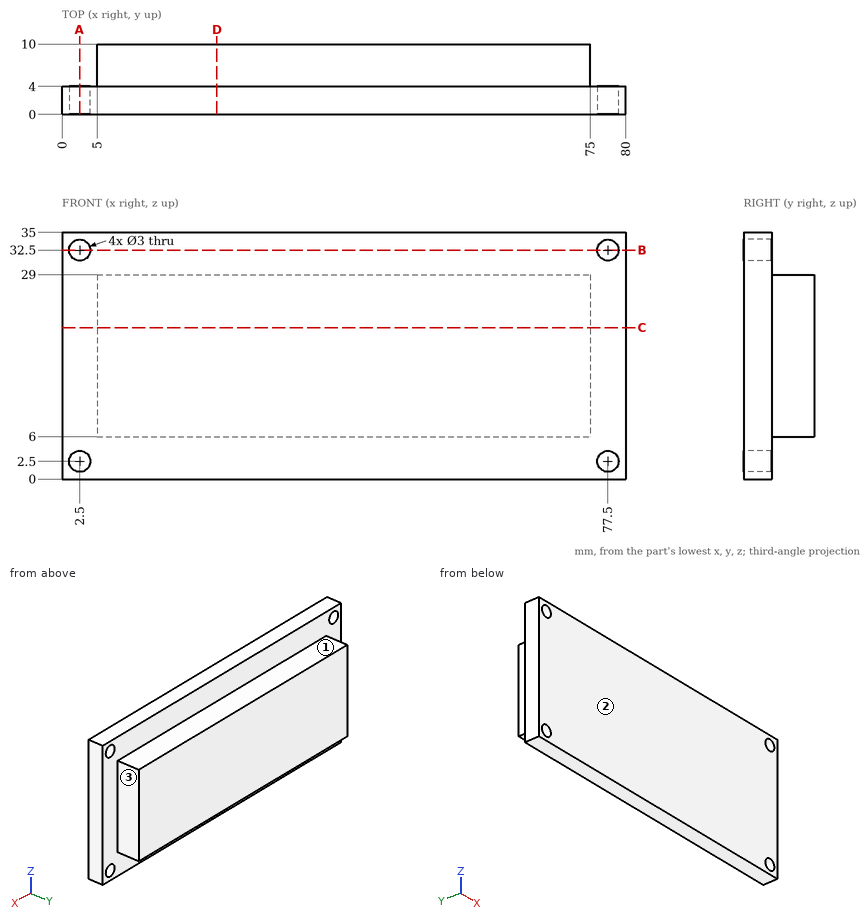
Print and shaded views of the part. All mm, measured from the part's lowest x, y and z. A direction names the side the tool comes from. Give positions to 0.01 mm unless a question says otherwise; leave off trailing zeros. Order: outer loops, then holes, each group sorted by start corner. A loop starts at its lowest first (then second) coordinate and runs counter-clockwise, first axis right, second up. Notation, with made-up numbers: (84, -14) - (136, -14) arc R18 cw to (136, 10) - close; hole circle Ø4 at (68.25, -15.5). An arc over 180 degrees is marked (long way). One line per item, written item: value.
Item 1: Slice it at D-D (x = 22). List the corners of the cut face in (y, z), then the cut area to 3 significant figures.
Response values:
outline: (0, 0) - (4, 0) - (4, 6) - (10, 6) - (10, 29) - (4, 29) - (4, 35) - (0, 35) - close
area: 278 mm2
Item 2: Slice it at A-A (x = 2.5). List the corners of the cut face in (y, z).
Response values:
outline: (0, 0) - (4, 0) - (4, 1) - (0, 1) - close; (0, 4) - (4, 4) - (4, 31) - (0, 31) - close; (0, 34) - (4, 34) - (4, 35) - (0, 35) - close
Item 3: Pin check, flat tips, straight feed: pin 1 Ø3.5 at (x, z) = (77.5, 32.5) entering from +Y; pin 2 Ø1 at (x, y) = (54.5, 6.5) entering from -Z; pin 3 Ø2.5 at (x, z) = (2.5, 2.5) entering from -Y; pin 4 Ø4 at (x, y) = (23, 7.5) entering from +Z. Stop position of each tip, or through.
Response values:
pin 1: y = 4
pin 2: z = 6
pin 3: through
pin 4: z = 29
Item 4: Tool access for the marked faces 1, 2 and 3: list every direction of +Z, -Z, +X, -X, +Y, -Y with a clear straight run to the whole face (end or side of a thin tool).
Response values:
face 1: +Z, +X, -X, +Y
face 2: +Z, -Z, +X, -X, -Y
face 3: +Z, -Z, +X, +Y
Item 5: Slice it at B-B (z = 32.5). List the corners of the cut face in (x, y), then the cut area to 3 significant figures.
Response values:
outline: (0, 0) - (1, 0) - (1, 4) - (0, 4) - close; (4, 0) - (76, 0) - (76, 4) - (4, 4) - close; (79, 0) - (80, 0) - (80, 4) - (79, 4) - close
area: 296 mm2
Item 6: Slice it at C-C (z = 21.5). List the corners of the cut face in (x, y).
Response values:
outline: (0, 0) - (80, 0) - (80, 4) - (75, 4) - (75, 10) - (5, 10) - (5, 4) - (0, 4) - close
Item 7: Wall check: line 1 (X direction, y = 1.1, z = 32.5); line 2 (Z direction, x = 77.5, y = 2.9); line 3 (Z direction, x = 28, y = 8.5). Give the ranges that are in metal, low to high.
Response values:
line 1: 0 to 1, 4 to 76, 79 to 80
line 2: 0 to 1, 4 to 31, 34 to 35
line 3: 6 to 29
